Here's the drawing with two shaded views (mm, measured from the low corner). I have some questions. Coordinates: 2 decimals unless noted, no trailing zeros. Write each loop counter-clockwise with the first axis right and the second up, starting at its lowest first coordinate (ties: lowest second). Pieces come first, ordered by that corner, then holes.
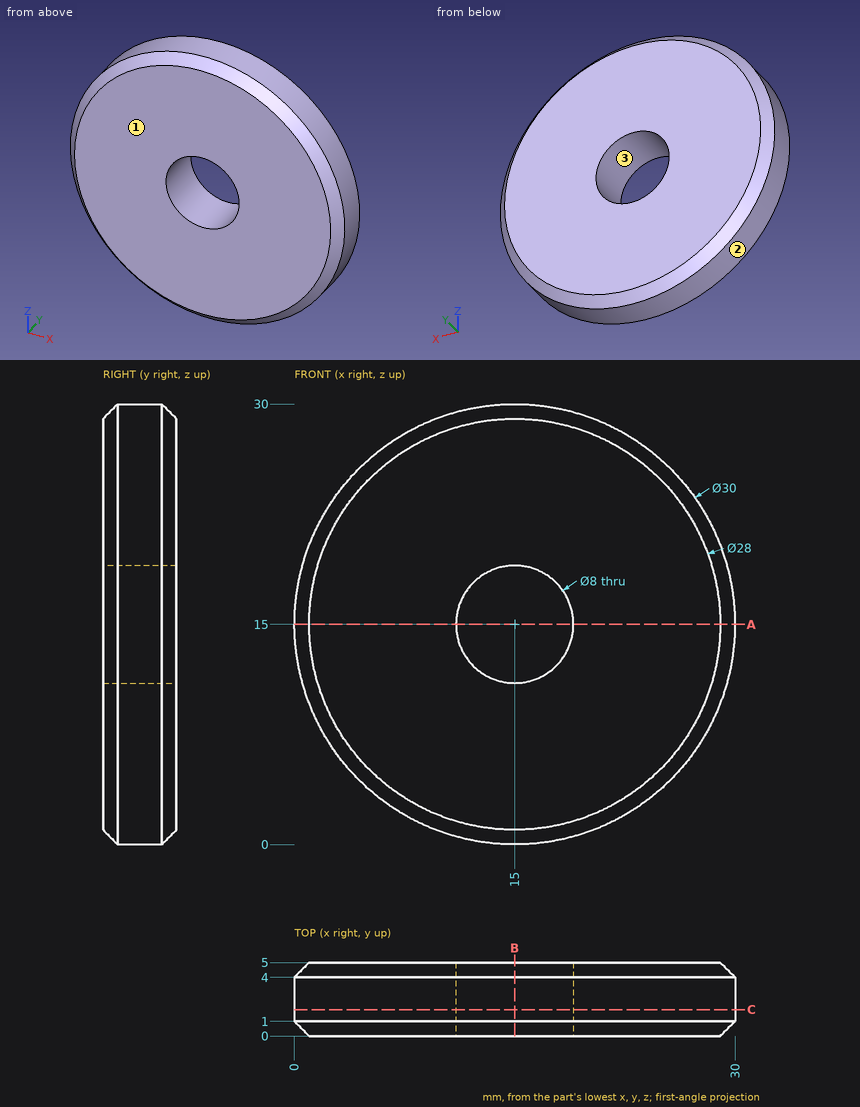
1. If we section it at A-A, the plane z = 15: List the corners of the cut face in (x, y) for me.
2. I'm going to push flat-ended pins straight in: P1, Ø2, axis at x = 8.5, y = 4.5, coming from the +Z side; P2, Ø2, axis at y = 1.5, z = 5.5, coming from the -X side; P3, Ø1.5, axis at x = 20.5, y = 2.5, coming from the +Z side. Where does each tip first touch, or does it pass through?
3. If we section it at C-C, the plane y = 1.8: List the corners of the cut face in (x, z) for me.
4. If we section it at B-B, the plane x = 15: List the corners of the cut face in (y, z) for me, plus the area to 3 significant figures.
5. We'd pull the mould along Z, two halves only. Please class the marked faces 1, 2 and 3: released by +Z, released by -Z, zero draft, split by the parting line, or undercut.
6. If I drill on L1, parallel to X at y = 3.6, z = 15; L2, parallel to X at y = 4.25, z = 15.5; L3, parallel to Z at x = 16, y = 3.3, over which ranges is the centre line in solid material (lowest first)?
Answers:
1. outline: (0, 1) - (1, 0) - (11, 0) - (11, 5) - (1, 5) - (0, 4) - close; (19, 0) - (29, 0) - (30, 1) - (30, 4) - (29, 5) - (19, 5) - close
2. P1: stops at z = 28.9
2. P2: stops at x = 2.64
2. P3: stops at z = 29.23
3. outline: circle Ø30 at (15, 15); hole circle Ø8 at (15, 15)
4. outline: (0, 1) - (1, 0) - (4, 0) - (5, 1) - (5, 11) - (0, 11) - close; (0, 19) - (5, 19) - (5, 29) - (4, 30) - (1, 30) - (0, 29) - close
4. area: 108 mm2
5. face 1: zero draft
5. face 2: split by the parting line
5. face 3: undercut
6. L1: x = 0 to 11, 19 to 30
6. L2: x = 0.26 to 11.03, 18.97 to 29.74
6. L3: z = 0.03 to 11.13, 18.87 to 29.97
